For this review, take the finished solid that the model builds, in its own axes (mm). Face numbers are marked on the shaded views. A direction names the side the tool comes from. Give positions to 0.01 mm unless a question says otherwise; leave off trailing zeros. Write each loop counter-clockwise with the first axis right and the second up, starting at its lowest first coordinate (ties: lowest second). Pieces come first, ordered by that corner, then holes. Notation, with made-up numbers: (-4.5, -30) -> (17.5, -30) arc R31 cw to (17.5, -3) -> close; hole circle Ø2 at (-31.5, 48.5). An arc over 180 degrees is marked (long way). Return JSON: item names as keys, results as strings.
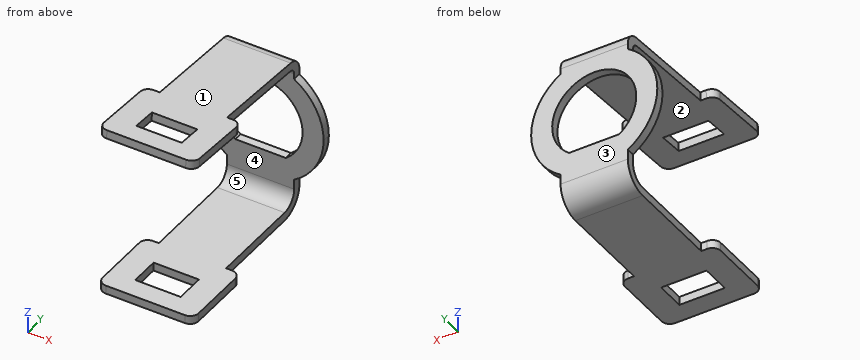
from build123d import *

# Parameters (mm, degrees)
PAD048_DEPTH    = 7.5
SKETCH077_W     = 3.5
SKETCH077_H     = 5.4
POCKET022_DEPTH = 1
SKETCH078_W     = 3
SKETCH078_H     = 5.4
POCKET023_DEPTH = 1
POCKET024_DEPTH = 3
FILLET020_R     = 1


with BuildPart() as part:
    # Sketch076 → Pad048 (new body, symmetric)
    with BuildSketch(Plane.YZ):
        with BuildLine():
            Line((25, -7.5500986951), (25, 7))
            ThreePointArc((25, 7), (24.786034319, 7.5445766952), (24.2585905577, 7.7978515818))
            Line((24.2585905577, 7.7978515818), (3.1155236405, 9.3505013609))
            Line((3.1155236405, 9.3505013609), (3.1887618377, 10.3478158381))
            Line((3.1887618377, 10.3478158381), (24.3318287548, 8.795166059))
            ThreePointArc((26, 7), (25.5185772178, 8.2252975641), (24.3318287548, 8.795166059))
            Line((26, 7), (26, -7.5500986951))
            ThreePointArc((23.1706790045, -10.3499451694), (25.1695051679, -9.540337222), (26, -7.5500986951))
            Line((2.9717865833, -10.1384151302), (23.1706790045, -10.3499451694))
            Line((2.9822583674, -9.1384699609), (2.9717865833, -10.1384151302))
            Line((23.1811507886, -9.35), (2.9822583674, -9.1384699609))
            ThreePointArc((23.1811507886, -9.35), (24.4661104651, -8.8295377481), (25, -7.5500986951))
        make_face()
    extrude(amount=PAD048_DEPTH, both=True)

    # Sketch077 (on Face10 of Pad048) → Pocket022 (cut)
    with BuildSketch(Plane(origin=(0, -0.1058355924, -10.106185168), x_dir=(0, 0.9999451694, -0.0104717841), z_dir=(0, -0.0104717841, -0.9999451694))):
        Polygon((3.0777909329, -5.7), (12.0777909329, -5.7), (12.0777909329, -4), (26.0777909329, -4), (26.0777909329, -7.5), (3.0777909329, -7.5), align=None)
        Polygon((3.0777909329, 5.7), (12.0777909329, 5.7), (12.0777909329, 4), (26.0777909329, 4), (26.0777909329, 7.5), (3.0777909329, 7.5), align=None)
        with Locations((7.2277909329, 0)):
            Rectangle(SKETCH077_W, SKETCH077_H)
    extrude(amount=-POCKET022_DEPTH, mode=Mode.SUBTRACT)

    # Sketch078 (on Face23 of Pocket022) → Pocket023 (cut)
    with BuildSketch(Plane(origin=(0, 0.7729241259, 10.52522387), x_dir=(0, -0.9973144772, 0.0732381971), z_dir=(0, 0.0732381971, 0.9973144772))):
        Polygon((-2.4223429689, 7.5), (-25.4223429689, 7.5), (-25.4223429689, 4), (-11.4223429689, 4), (-11.4223429689, 5.7), (-2.4223429689, 5.7), align=None)
        Polygon((-2.4223429689, -7.5), (-25.4223429689, -7.5), (-25.4223429689, -4), (-11.4223429689, -4), (-11.4223429689, -5.7), (-2.4223429689, -5.7), align=None)
        with Locations((-6.3223429689, 0)):
            Rectangle(SKETCH078_W, SKETCH078_H)
    extrude(amount=-POCKET023_DEPTH, mode=Mode.SUBTRACT)

    # Sketch079 (on Face21 of Pocket023) → Pocket024 (cut)
    with BuildSketch(Plane.ZX.offset(26)):
        with BuildLine():
            ThreePointArc((-6.3442887702, -4), (-3.6228442441, -6.5669627366), (-1.314e-07, -7.5))
            Line((-9.3724594748, -7.5), (-1.314e-07, -7.5))
            Line((-9.3724594748, -4), (-9.3724594748, -7.5))
            Line((-9.3724594748, -4), (-6.3442887702, -4))
        make_face()
        with BuildLine():
            ThreePointArc((3.60745e-05, -7.4999999999), (3.6228599799, -6.5669540554), (6.3442887702, -4))
            Line((9.3724594748, -4), (6.3442887702, -4))
            Line((9.3724594748, -4), (9.3724594748, -7.4999999999))
            Line((9.3724594748, -7.4999999999), (3.60745e-05, -7.4999999999))
        make_face()
        with BuildLine():
            ThreePointArc((-3.60745e-05, 7.4999999999), (-3.6228599799, 6.5669540554), (-6.3442887702, 4))
            Line((-9.3724594748, 4), (-6.3442887702, 4))
            Line((-9.3724594748, 4), (-9.3724594748, 7.4999999999))
            Line((-9.3724594748, 7.4999999999), (-3.60745e-05, 7.4999999999))
        make_face()
        with BuildLine():
            ThreePointArc((6.3442887702, 4), (3.6228599799, 6.5669540554), (3.60745e-05, 7.4999999999))
            Line((9.3724594748, 7.4999999999), (3.60745e-05, 7.4999999999))
            Line((9.3724594748, 4), (9.3724594748, 7.4999999999))
            Line((9.3724594748, 4), (6.3442887702, 4))
        make_face()
        with BuildLine():
            ThreePointArc((-4, -3), (5, 0), (-4, 3))
            Line((-4, 3), (-4, -3))
        make_face()
    extrude(amount=-POCKET024_DEPTH, mode=Mode.SUBTRACT)

    # Fillet020
    fillet020_edges = [part.edges().sort_by_distance(p)[0] for p in [
        (5.7, 2.977022, -9.638443),
        (-5.7, 2.977022, -9.638443),
        (5.7, 3.152143, 9.849159),
        (-5.7, 3.152143, 9.849159),
        (-5.7, 12.127973, 9.190015),
        (5.7, 12.127973, 9.190015),
        (5.7, 11.976529, -9.732689),
        (-5.7, 11.976529, -9.732689),
    ]]
    fillet(fillet020_edges, radius=FILLET020_R)


with BuildPart() as part_1:
    # Body027 placement: moved
    add(part.part.moved(Location((0, 25.7, 0))))


solid = part_1.part
1. For the marked faces 4 and 5, list the 3-axis set-ups (+Z, -Z, +X, -X, +Y, -Y) from which the entire face can be reached by the end or side of a thin tool; tool diameter is ignored.
Results found:
{"face 4": "+X, -X, -Y", "face 5": "+X, -X"}
2. Add section D-D, the plane z = -1.5. State the section outline as (x, y) points.
Results found:
{"outline": "(-7.35, 50.7) -> (-4.77, 50.7) -> (-4.77, 51.7) -> (-7.35, 51.7) -> close; (4.77, 50.7) -> (7.35, 50.7) -> (7.35, 51.7) -> (4.77, 51.7) -> close"}
3. For pin 1 (1 mm diameter, centred on y = 31, z = -8, fed in from +X); pin 2 (1.7 mm diameter, centred on y = 44.5, z = 8, fed in from -X); pin 3 (6 mm diameter, centred on x = 0, z = -6, fed in from -Y); pin 4 (0.5 mm diameter, centred on y = 33.5, z = -9.5, fed in from +X), all flat-tipped, find the tip position at first contact; note any pin that passes through.
Results found:
{"pin 1": "passes through", "pin 2": "stops at x = -4", "pin 3": "stops at y = 49.97", "pin 4": "stops at x = 5.7"}
4. Add section C-C, the plane z = 2.25. State the section outline as (x, y) points.
Results found:
{"outline": "(-7.15, 50.7) -> (-4.47, 50.7) -> (-4.47, 51.7) -> (-7.15, 51.7) -> close; (4.47, 50.7) -> (7.15, 50.7) -> (7.15, 51.7) -> (4.47, 51.7) -> close"}
5. To check wall thickness, follow probe 1 along X at (y, z) = (51.15, 0); probe 2 along Y at (x, z) = (5.5, -3.5); probe 3 along Z at (x, y) = (-1, 37). State the ranges of each line that lie inside material, in increasing order.
Results found:
{"probe 1": "x = -7.5 to -5, 5 to 7.5", "probe 2": "y = 50.7 to 51.7", "probe 3": "z = -10.23 to -9.23, 8.75 to 9.75"}
6. The part is to be moulded in two halves that separate along Z. For the marked faces 1, 2 and 3, say which applies: +Z half, -Z half, draft (parallel to the pull), parting line (faces both ways), or undercut.
Results found:
{"face 1": "+Z half", "face 2": "undercut", "face 3": "draft"}
7. Add section B-B, the plane y = 33. State the section outline as (x, z) points, plus the area to 3 significant figures.
Results found:
{"outline": "(-5.7, -10.18) -> (-2.7, -10.18) -> (-2.7, -9.18) -> (-5.7, -9.18) -> close; (-5.7, 9.04) -> (-2.7, 9.04) -> (-2.7, 10.05) -> (-5.7, 10.05) -> close; (2.7, -10.18) -> (5.7, -10.18) -> (5.7, -9.18) -> (2.7, -9.18) -> close; (2.7, 9.04) -> (5.7, 9.04) -> (5.7, 10.05) -> (2.7, 10.05) -> close", "area": "12.0 mm²"}
8. Add section A-A, the plane x = 0. State the section outline as (y, z) points, plus the area to 3 significant figures.
Results found:
{"outline": "(28.67, -10.14) -> (31.07, -10.16) -> (31.08, -9.16) -> (28.68, -9.14) -> close; (28.82, 9.35) -> (31.21, 9.17) -> (31.28, 10.17) -> (28.89, 10.35) -> close; (34.2, 8.96) -> (49.96, 7.8) arc R0.8 cw to (50.7, 7) -> (50.7, 5) -> (51.7, 5) -> (51.7, 7) arc R1.8 ccw to (50.03, 8.8) -> (34.27, 9.95) -> close; (34.57, -10.2) -> (48.87, -10.35) arc R2.8 ccw to (51.7, -7.55) -> (51.7, -4) -> (50.7, -4) -> (50.7, -7.55) arc R1.8 cw to (48.88, -9.35) -> (34.58, -9.2) -> close", "area": "46.0 mm²"}
